from build123d import *

# Parameters (mm, degrees)
SKETCH_1_W          = 40
SKETCH_1_H          = 20
EXTRUDE_1_DEPTH     = 20
SKETCH_2_W          = 8
SKETCH_2_H          = 4
EXTRUDE_2_DEPTH     = 10
CUT_EXTRUDE_8_DEPTH = 20
SKETCH_13_R         = 1
EXTRUDE_5_DEPTH     = 8
CUT_EXTRUDE_9_DEPTH = 20


with BuildPart() as part:
    # 草图1 → 凸台-拉伸1 (new body)
    with BuildSketch(Plane(origin=(0, 0, 0), x_dir=(1, 0, 0), z_dir=(0, 1, 0))):
        with Locations((18, 0)):
            Rectangle(SKETCH_1_W, SKETCH_1_H)
    extrude(amount=EXTRUDE_1_DEPTH)

    # 草图2 → 凸台-拉伸2 (add)
    with BuildSketch(Plane.ZY.offset(2)):
        with Locations((0, 2)):
            Rectangle(SKETCH_2_W, SKETCH_2_H)
    extrude(amount=EXTRUDE_2_DEPTH)

    # 草图12 → 切除-拉伸8 (cut)
    with BuildSketch(Plane.XY.offset(4)):
        with BuildLine():
            Line((-5, 2), (-18.474771325, 2))
            Line((-18.474771325, 2), (-18.474771325, 0))
            Line((-18.474771325, 0), (-5, 0))
            ThreePointArc((-5, 0), (-6, 1), (-5, 2))
        make_face()
    extrude(amount=-CUT_EXTRUDE_8_DEPTH, mode=Mode.SUBTRACT)

    # 草图13 → 凸台-拉伸5 (add)
    with BuildSketch(Plane.XY.offset(4)):
        with Locations((-12, 3)):
            Circle(SKETCH_13_R)
    extrude(amount=-EXTRUDE_5_DEPTH)

    # 草图14 → 切除-拉伸9 (cut)
    with BuildSketch(Plane.XY.offset(10)):
        Polygon((40.736846826, 20.947387303), (-2, 20), (-2, 15), (7.959394399, 15.0101514), (17.918788798, 10.020302801), (27.939091598, 0), (43.275764459, 0), align=None)
    extrude(amount=-CUT_EXTRUDE_9_DEPTH, mode=Mode.SUBTRACT)


solid = part.part
Can you work these out from the model? Positions are in its coordinate system, mm. A direction names the side the tool comes from. Round coordinates to 2 decimals unless told otherwise and drop trailing zeros. Loops run counter-clockwise (first coordinate to the right, second up) from the corner with the lowest first, then second, coordinate; pieces in that order, holes last. Notation, with made-up numbers: (89, 73) - (125, 73) arc R21 cw to (125, 104) - close; hole circle Ø11 at (-33.75, 27). An arc over 180 degrees is marked (long way). Write item = value, one per line. Start each with the question number.
(1) For faces 5 (the face through (-6.2, 2.4, 4)), 6 (the face through (12.87, 12.55, 0.14)), 7 (the face through (-6.4, 2.5, -4)), which set-ups out of +Z, -Z, +X, -X, +Y, -Y let a thin tool reach every point of the face, with its end or its side?
(2) If we section it at C-C (x = -7.5): Please give me the cut outline in (y, z).
(3) If I drill on probe 1 along Y at (x, z) = (-0.5, 9); probe 2 along Y at (x, z) = (-9, 3.5); probe 3 along Z at (x, y) = (-6, 3.75), over which ranges is the centre line in solid material (lowest first)? Write a range as [from, to].
(4) If we section it at A-A (z = 0.25): Please give me the cut outline in (x, y), and give its area (3 significant figures).
(5) If we section it at D-D (z = 7.75): Please give me the cut outline in (x, y), and give its area (3 significant figures).
(6) For P1, Ø8, axis at x = 12.5, z = 1, coming from the -Y side; P2, Ø3, axis at y = 5.5, z = 4.5, coming from the -X side; P3, Ø1.2, axis at x = -7.5, y = 3, coming from the +Z side; P4, Ø8, axis at x = 22.5, z = -7.5, coming from the +Y side, each with a flat end and sliding along its axis, tell me the tip position at first contact or that it passes through.
(7) If we section it at B-B (y = 2.5): Please give me the cut outline in (x, z).
(8) If we mould it in two halves opening along Y, with no side actions, what happens to faces 1 (the face through (9, 6, 10)), 2 (the face through (-6, 1, 0)), 3 (the face through (-13, 3, 0)), 4 (the face through (-7, 4, 0))? For each: released by +Y, released by -Y, zero draft, split by the parting line, or undercut.
Ans:
q1.face_5 = +Z, -X, +Y, -Y
q1.face_6 = +Z, -Z, +X, +Y
q1.face_7 = -Z, -X, +Y, -Y
q2.outline = (2, -4) - (4, -4) - (4, 4) - (2, 4) - close
q3.probe_1 = [0, 15]
q3.probe_2 = [2, 4]
q3.probe_3 = [-4, 4]
q4.outline = (-12, 2) - (-5, 2) arc R1 ccw to (-5, 0) - (27.94, 0) - (17.92, 10.02) - (7.96, 15.01) - (-2, 15) - (-2, 4) - (-12, 4) arc R1 ccw to start
q4.area = 353 mm²
q5.outline = (-2, 0) - (27.94, 0) - (17.92, 10.02) - (7.96, 15.01) - (-2, 15) - close
q5.area = 324 mm²
q6.P1 = 0
q6.P2 = -2
q6.P3 = 4
q6.P4 = 9.44
q7.outline = (-12.87, -4) - (-2, -4) - (-2, -10) - (25.44, -10) - (25.44, 10) - (-2, 10) - (-2, 4) - (-12.87, 4) - close
q8.face_1 = zero draft
q8.face_2 = undercut
q8.face_3 = split by the parting line
q8.face_4 = released by +Y
